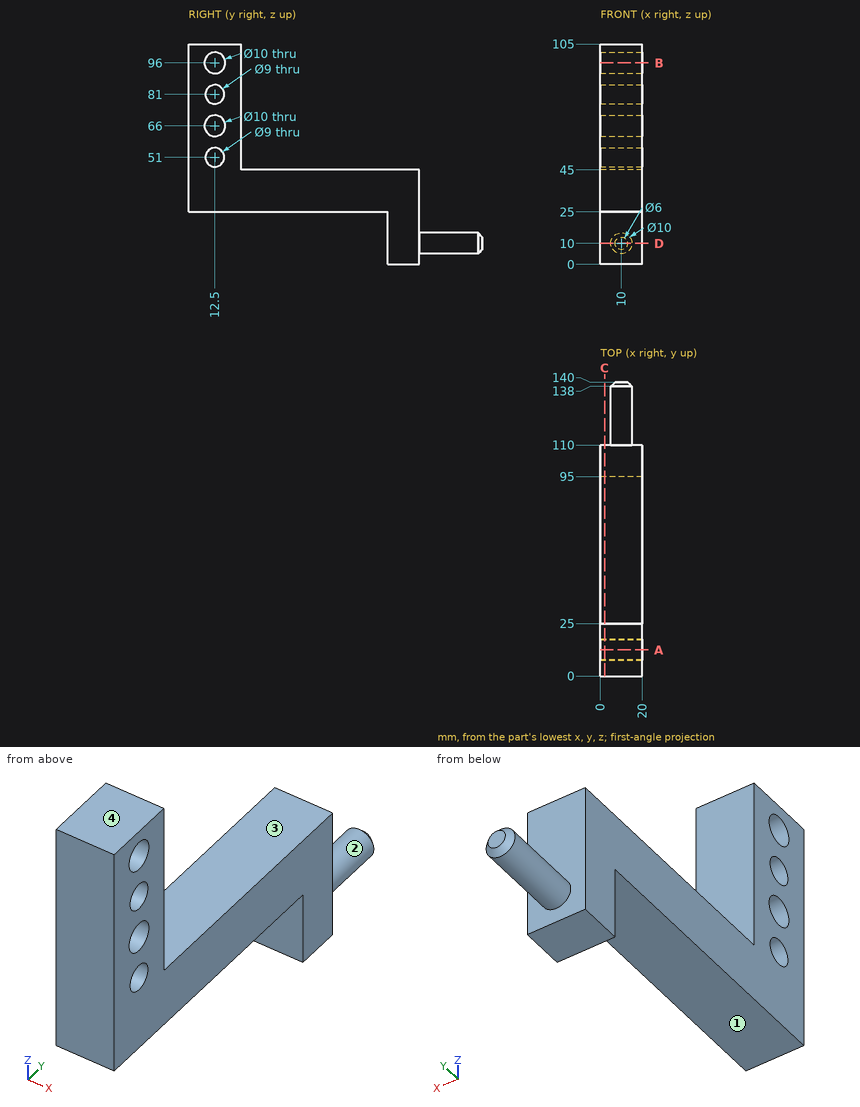
Input: dimensioned drawing with shaded views. Units: mm. Origin: part minimum x, y, z. A direction names the side the tool comes from. Round coordinates to 2 decimals unless told otherwise and drop trailing zeros. Loops run counter-clockwise (first coordinate to the right, second up) from the corner with the lowest first, then second, coordinate; pieces in that order, holes last. Notation, with made-up numbers: M 82.25,8.5 L 118.25,8.5 A37 cw 118.25,47.5 Z; hole C 39.5,-5.75 d2. An arc over 180 degrees is marked long. Return JSON: item names as keys, results as strings. Group by question number.
1. Section query B-B on z = 96. Output: boundary loops of the cut face in (x, y), and give its area (3 significant figures).
2. Pin query (flat end, axial travel): pin 1 (12 mm diameter, centred on x = 6.5, z = 47, fed in from +Y); pin 2 (10 mm diameter, centred on x = 14, z = 85, fed in from +Y); pin 3 (10.5 mm diameter, centred on y = 12.5, z = 51, fed in from -X); pin 4 (10 mm diameter, centred on x = 16, y = 101, fed in from +Z). Return the tip coordinate at first contact, or that it passes through.
3. Section query D-D on z = 10. Output: boundary loops of the cut face in (x, y), and give its area (3 significant figures).
4. Material intervals for line 1 along Z through (x, y) = (11.25, 12.5); line 2 along Y through (x, z) = (9.5, 38); line 3 along Z through (x, y) = (18, 20), sorted ascending. Write a range as from..to.
5. Section query C-C on x = 2. Output: boundary loops of the cut face in (y, z).
6. Section query A-A on y = 12.5. Output: boundary loops of the cut face in (x, z), and give its area (3 significant figures).
7. Reachability of the marked faces 1, 2, 3 and 4 from +Z, -Z, +X, -X, +Y, -Y: full face, straight path, thin tool, end or side. Return the list, or none.
Checks:
{
 "1": {"outline": "M 0,0 L 20,0 L 20,7.5 L 0,7.5 Z; M 0,17.5 L 20,17.5 L 20,25 L 0,25 Z", "area": "300 mm²"},
 "2": {"pin 1": "stops at y = 110", "pin 2": "stops at y = 25", "pin 3": "stops at x = 0", "pin 4": "stops at z = 45"},
 "3": {"outline": "M 0,95 L 20,95 L 20,110 L 15,110 L 15,138 L 13,140 L 7,140 L 5,138 L 5,110 L 0,110 Z", "area": "596 mm²"},
 "4": {"line 1": "z = 25..46.5, 55.5..61, 71..76.5, 85.5..91, 101..105", "line 2": "y = 0..110", "line 3": "z = 25..105"},
 "5": {"outline": "M 0,25 L 95,25 L 95,0 L 110,0 L 110,45 L 25,45 L 25,105 L 0,105 Z; hole C 12.5,66 d10; hole C 12.5,96 d10; hole C 12.5,51 d9; hole C 12.5,81 d9"},
 "6": {"outline": "M 0,25 L 20,25 L 20,46.5 L 0,46.5 Z; M 0,55.5 L 20,55.5 L 20,61 L 0,61 Z; M 0,71 L 20,71 L 20,76.5 L 0,76.5 Z; M 0,85.5 L 20,85.5 L 20,91 L 0,91 Z; M 0,101 L 20,101 L 20,105 L 0,105 Z", "area": "840 mm²"},
 "7": {"face 1": "-Z, +X, -X, -Y", "face 2": "+Y", "face 3": "+Z, +X, -X, +Y", "face 4": "+Z, +X, -X, +Y, -Y"}
}
